```python
from build123d import *

# Parameters (mm, degrees)
F2_R     = 9.5
F3_DEPTH = 12.7
F4_R     = 8
F5_DEPTH = 1.5
F7_DEPTH = 12.7


# Not quite as in the source:
# - ends of sketch curves that miss each other by under 0.0002 mm in the source are joined
# - a feature names something its author has since deleted; it is built from what else it names


with BuildPart() as f1:
    # F0 (on Front) → F1 (revolve)
    with BuildSketch(Plane.XZ):
        with BuildLine():
            ThreePointArc((-12, -12.5), (-8.4852813742, -20.9852813742), (0, -24.5))
            Line((0, -24.5), (0, -12.5))
            Line((0, -12.5), (-12, -12.5))
        make_face()
        with BuildLine():
            Line((-12, -12.5), (0, -12.5))
            Line((0, -12.5), (0, 0))
            Line((0, 0), (-9, 0))
            ThreePointArc((-9, 0), (-11.177394056, -6.0874254266), (-12, -12.5))
        make_face()
    revolve(axis=Axis((0, 0, -12.25), (0, 0, 1)))

    # F2 (on Front) → F3 (cut, symmetric)
    with BuildSketch(Plane.XZ):
        with Locations((0, -12.25)):
            Circle(F2_R)
    extrude(amount=F3_DEPTH, both=True, mode=Mode.SUBTRACT)

    # F4 (on Top) → F5 (cut)
    with BuildSketch(Plane.XY):
        Circle(F4_R)
        with BuildLine():
            ThreePointArc((-1.9356951783, -3.7273427769), (-3.58956263, -2.1806054493), (-4.2, 0))
            ThreePointArc((-4.2, 0), (-3.58956263, 2.1806054493), (-1.9356951783, 3.7273427769))
            Line((-1.9356951783, 3.7273427769), (-4.191, 3.7254119238))
            Line((-4.191, 3.7254119238), (-4.191, 5.729))
            Line((-4.191, 5.729), (0, 5.729))
            Line((0, 5.729), (4.191, 5.7290075347))
            Line((4.191, 5.7290075347), (4.191, 3.7289706524))
            Line((4.191, 3.7289706524), (1.9325573402, 3.7289706524))
            ThreePointArc((1.9325573402, 3.7289706524), (3.5886446487, 2.1821158506), (4.2, 0))
            ThreePointArc((4.2, 0), (3.58956263, -2.1806054493), (1.9356951783, -3.7273427769))
            Line((1.9356951783, -3.7273427769), (4.3272348121, -3.7273427769))
            Line((4.3272348121, -3.7273427769), (4.3272348121, -5.7290102))
            Line((4.3272348121, -5.7290102), (0, -5.7290102))
            Line((0, -5.7290102), (-4.191, -5.7290102))
            Line((-4.191, -5.7290102), (-4.191, -3.7273427769))
            Line((-4.191, -3.7273427769), (-1.9356951783, -3.7273427769))
        make_face(mode=Mode.SUBTRACT)
        with BuildLine():
            ThreePointArc((-2.32, 0), (0, -2.32), (2.32, 0))
            ThreePointArc((2.32, 0), (0, 2.32), (-2.32, 0))
        make_face()
    extrude(amount=-F5_DEPTH, mode=Mode.SUBTRACT)

    # F6 (on Right) → F7 (cut, symmetric)
    with BuildSketch(Plane.YZ):
        with BuildLine():
            Line((3.5, -9.3865861699), (3.5, -26.5))
            Line((3.5, -26.5), (11.7441575179, -26.5))
            Line((11.7441575179, -26.5), (11.7441575179, -12.5))
            Line((11.7441575179, -12.5), (11.7441575179, -2.5))
            Line((11.7441575179, -2.5), (10.2463875179, -2.5))
            ThreePointArc((10.2463875179, -2.5), (6.0394031611, -5.1264769814), (3.5, -9.3865861699))
        make_face()
    extrude(amount=F7_DEPTH, both=True, mode=Mode.SUBTRACT)


solid = f1.part
```
Part model, mm, in its own coordinate system. A direction names the side the tool comes from. Coordinates: 2 decimals unless noted, no trailing zeros. Order: outer loops, then holes, each group sorted by start corner. A loop starts at its lowest first (then second) coordinate and runs counter-clockwise, first axis right, second up. Notation, with made-up numbers: (82, -38) -> (127, -38) arc R23 cw to (127, -27) -> close; hole circle Ø11 at (43.5, 84.25). An arc over 180 degrees is marked (long way). Put each result on its own line as item: value. Start each with the question number.
(1) Band-saw the part on B-B (z = -13.75). Give the cut face in (x, y), then the cut area to 3 significant figures.
(2) Mould opens along X. For faces 3 (the face through (3, 3.729, -1)), 4 (the face through (-1, 3.5, -22)), 5 (the face through (3.4, -3.4, -1.5)) say: pulls with the +X half, pulls with the -X half, needs draft (parallel to the pull), parting line crosses it, or undercut.
(3) Probe line 1 along Y through (x, z) = (0, -0.75); line 2 along Z through (x, y) = (0, -3.5); line 3 along Z through (x, y) = (0, -5.25). List the from-to ranges inside material, lowest first. Write a range as [from, to].
(4) Pin check, flat tips, straight feed: pin 1 Ø2 at (x, z) = (-0.5, -20.5) entering from +Y; pin 2 Ø1.4 at (x, y) = (-0.5, -0.5) entering from +Z; pin 3 Ø0.8 at (x, z) = (3.5, -1) entering from -Y; pin 4 Ø1.2 at (y, z) = (5, -1) entering from +X. Stop position of each tip, or through.
(5) Band-saw the part on A-A (z = -20.75). Give the cut face in (x, y), then the cut area to 3 significant figures.
(6) Which spindle directions (+Z, -Z, +X, -X, +Y, -Y) get a long thin tool onto all of the face, cutting with end or side? Do faces 1 (the face through (-1.73, -7.81, -0.74)), 2 (the face through (0, -3, 0)). Say none if no direction does.
Determined:
1. outline: (-11.41, 3.5) arc R11.93 ccw to (-9.38, -7.38) -> (-9.38, 3.5) -> close; (9.38, -7.38) arc R11.93 ccw to (11.41, 3.5) -> (9.38, 3.5) -> close
1. area: 42.4 mm²
2. face 3: undercut
2. face 4: needs draft
2. face 5: undercut
3. line 1: y = [-9.35, -8], [-5.73, -2.32], [2.32, 5.73], [8, 9.35]
3. line 2: z = [-23.98, -21.75], [-2.75, 0]
3. line 3: z = [-23.29, -21.75], [-2.75, 0]
4. pin 1: passes through
4. pin 2: stops at z = -1.5
4. pin 3: stops at y = -9.03
4. pin 4: stops at x = 8.49
5. outline: (-7.98, 3.5) arc R8.71 ccw to (-4.24, -7.61) -> (-4.24, 3.5) -> close; (4.24, -7.61) arc R8.71 ccw to (7.98, 3.5) -> (4.24, 3.5) -> close
5. area: 78.0 mm²
6. face 1: +Z
6. face 2: +Z, +X, -X, +Y, -Y
